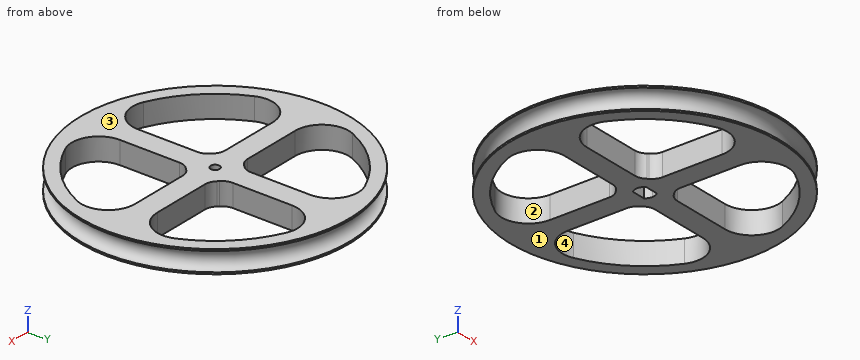
```python
from build123d import *

# Parameters (mm, degrees)
BOSS_EXTRUDE1_START = -6.35
SKETCH3_W           = 6.35
SKETCH3_H           = 6.35
BOSS_EXTRUDE1_DEPTH = 6.35
FILLET1_R           = 7.62
FILLET2_R           = 3.81
BOSS_EXTRUDE2_START = -1.5875
SKETCH4_R           = 1.27
BOSS_EXTRUDE2_DEPTH = 1.5875


with BuildPart() as part:
    # Sketch2 → Revolve1 (revolve)
    with BuildSketch(Plane(origin=(0, 0, 0), x_dir=(1, 0, 0), z_dir=(0, 1, 0))):
        with BuildLine():
            ThreePointArc((38.1, 2.667), (35.433, 0), (38.1, -2.667))
            Line((38.1, -2.667), (38.1, -3.175))
            Line((38.1, -3.175), (34.29, -3.175))
            Line((34.29, -3.175), (34.29, 3.175))
            Line((34.29, 3.175), (38.1, 3.175))
            Line((38.1, 3.175), (38.1, 2.667))
        make_face()
    revolve(axis=Axis((0, 0, 2.667), (0, 0, -1)))

    # Sketch3 → Boss-Extrude1 (add)
    # profile 1 of 19: a face of its own
    with BuildSketch(Plane.XY.offset(3.175).offset(BOSS_EXTRUDE1_START)):
        with BuildLine():
            ThreePointArc((-34.142692849, 3.175), (-34.29, 0), (-34.142692849, -3.175))
            Line((-34.142692849, -3.175), (-5.645432136, -3.175))
            ThreePointArc((-5.645432136, -3.175), (-6.477, 0), (-5.645432136, 3.175))
            Line((-5.645432136, 3.175), (-34.142692849, 3.175))
        make_face()
    # profile 2 of 19: a face of its own
    with BuildSketch(Plane.XY.offset(3.175).offset(BOSS_EXTRUDE1_START)):
        with BuildLine():
            Line((5.645432136, -3.175), (34.142692849, -3.175))
            ThreePointArc((34.142692849, -3.175), (34.253153415, -1.589207695), (34.29, 0))
            ThreePointArc((34.29, 0), (34.253153415, 1.589207695), (34.142692849, 3.175))
            Line((34.142692849, 3.175), (5.645432136, 3.175))
            ThreePointArc((5.645432136, 3.175), (6.265660099, 1.641046169), (6.477, 0))
            ThreePointArc((6.477, 0), (6.265660099, -1.641046169), (5.645432136, -3.175))
        make_face()
    # profile 3 of 19: a face of its own
    with BuildSketch(Plane.XY.offset(3.175).offset(BOSS_EXTRUDE1_START)):
        with BuildLine():
            ThreePointArc((-5.645432136, 3.175), (-6.477, 0), (-5.645432136, -3.175))
            Line((-5.645432136, -3.175), (-3.175, -3.175))
            Line((-3.175, -3.175), (-3.175, 3.175))
            Line((-3.175, 3.175), (-5.645432136, 3.175))
        make_face()
    # profile 4 of 19: a face of its own
    with BuildSketch(Plane.XY.offset(3.175).offset(BOSS_EXTRUDE1_START)):
        with BuildLine():
            Line((-3.175, 5.645432136), (-3.175, 3.175))
            Line((-3.175, 3.175), (3.175, 3.175))
            Line((3.175, 3.175), (3.175, 5.645432136))
            ThreePointArc((3.175, 5.645432136), (0, 6.477), (-3.175, 5.645432136))
        make_face()
    # profile 5 of 19: a face of its own
    with BuildSketch(Plane.XY.offset(3.175).offset(BOSS_EXTRUDE1_START)):
        with BuildLine():
            Line((-3.175, -5.645432136), (-3.175, -34.142692849))
            ThreePointArc((-3.175, -34.142692849), (0, -34.29), (3.175, -34.142692849))
            Line((3.175, -34.142692849), (3.175, -5.645432136))
            ThreePointArc((3.175, -5.645432136), (0, -6.477), (-3.175, -5.645432136))
        make_face()
    # profile 6 of 19: a face of its own
    with BuildSketch(Plane.XY.offset(3.175).offset(BOSS_EXTRUDE1_START)):
        with BuildLine():
            ThreePointArc((3.175, 34.142692849), (0, 34.29), (-3.175, 34.142692849))
            Line((-3.175, 34.142692849), (-3.175, 5.645432136))
            ThreePointArc((-3.175, 5.645432136), (0, 6.477), (3.175, 5.645432136))
            Line((3.175, 5.645432136), (3.175, 34.142692849))
        make_face()
    # profile 7 of 19: a face of its own
    with BuildSketch(Plane.XY.offset(3.175).offset(BOSS_EXTRUDE1_START)):
        with BuildLine():
            ThreePointArc((-3.175, 5.645432136), (-4.579930622, 4.579930622), (-5.645432136, 3.175))
            Line((-5.645432136, 3.175), (-3.175, 3.175))
            Line((-3.175, 3.175), (-3.175, 5.645432136))
        make_face()
    # profile 8 of 19: a face of its own
    with BuildSketch(Plane.XY.offset(3.175).offset(BOSS_EXTRUDE1_START)):
        with BuildLine():
            Line((3.175, 5.645432136), (3.175, 3.175))
            Line((3.175, 3.175), (5.645432136, 3.175))
            ThreePointArc((5.645432136, 3.175), (4.579930622, 4.579930622), (3.175, 5.645432136))
        make_face()
    # profile 9 of 19: a face of its own
    with BuildSketch(Plane.XY.offset(3.175).offset(BOSS_EXTRUDE1_START)):
        with BuildLine():
            Line((3.175, 3.175), (3.175, -3.175))
            Line((3.175, -3.175), (5.645432136, -3.175))
            ThreePointArc((5.645432136, -3.175), (6.265660099, -1.641046169), (6.477, 0))
            ThreePointArc((6.477, 0), (6.265660099, 1.641046169), (5.645432136, 3.175))
            Line((5.645432136, 3.175), (3.175, 3.175))
        make_face()
    # profile 10 of 19: a face of its own
    with BuildSketch(Plane.XY.offset(3.175).offset(BOSS_EXTRUDE1_START)):
        with BuildLine():
            ThreePointArc((-34.142692849, 3.175), (-34.29, 0), (-34.142692849, -3.175))
            Line((-34.142692849, -3.175), (-5.645432136, -3.175))
            ThreePointArc((-5.645432136, -3.175), (-6.477, 0), (-5.645432136, 3.175))
            Line((-5.645432136, 3.175), (-34.142692849, 3.175))
        make_face()
    # profile 11 of 19: a face of its own
    with BuildSketch(Plane.XY.offset(3.175).offset(BOSS_EXTRUDE1_START)):
        with BuildLine():
            Line((5.645432136, -3.175), (34.142692849, -3.175))
            ThreePointArc((34.142692849, -3.175), (34.253153415, -1.589207695), (34.29, 0))
            ThreePointArc((34.29, 0), (34.253153415, 1.589207695), (34.142692849, 3.175))
            Line((34.142692849, 3.175), (5.645432136, 3.175))
            ThreePointArc((5.645432136, 3.175), (6.265660099, 1.641046169), (6.477, 0))
            ThreePointArc((6.477, 0), (6.265660099, -1.641046169), (5.645432136, -3.175))
        make_face()
    # profile 12 of 19: a face of its own
    with BuildSketch(Plane.XY.offset(3.175).offset(BOSS_EXTRUDE1_START)):
        with BuildLine():
            Line((-3.175, -5.645432136), (-3.175, -34.142692849))
            ThreePointArc((-3.175, -34.142692849), (0, -34.29), (3.175, -34.142692849))
            Line((3.175, -34.142692849), (3.175, -5.645432136))
            ThreePointArc((3.175, -5.645432136), (0, -6.477), (-3.175, -5.645432136))
        make_face()
    # profile 13 of 19: a face of its own
    with BuildSketch(Plane.XY.offset(3.175).offset(BOSS_EXTRUDE1_START)):
        with BuildLine():
            ThreePointArc((3.175, 34.142692849), (0, 34.29), (-3.175, 34.142692849))
            Line((-3.175, 34.142692849), (-3.175, 5.645432136))
            ThreePointArc((-3.175, 5.645432136), (0, 6.477), (3.175, 5.645432136))
            Line((3.175, 5.645432136), (3.175, 34.142692849))
        make_face()
    # profile 14 of 19: a face of its own
    with BuildSketch(Plane.XY.offset(3.175).offset(BOSS_EXTRUDE1_START)):
        with BuildLine():
            Line((3.175, -3.175), (-3.175, -3.175))
            Line((-3.175, -3.175), (-3.175, -5.645432136))
            ThreePointArc((-3.175, -5.645432136), (0, -6.477), (3.175, -5.645432136))
            Line((3.175, -5.645432136), (3.175, -3.175))
        make_face()
    # profile 15 of 19: a face of its own
    with BuildSketch(Plane.XY.offset(3.175).offset(BOSS_EXTRUDE1_START)):
        with BuildLine():
            Line((-3.175, -3.175), (-5.645432136, -3.175))
            ThreePointArc((-5.645432136, -3.175), (-4.579930622, -4.579930622), (-3.175, -5.645432136))
            Line((-3.175, -5.645432136), (-3.175, -3.175))
        make_face()
    # profile 16 of 19: a face of its own
    with BuildSketch(Plane.XY.offset(3.175).offset(BOSS_EXTRUDE1_START)):
        with BuildLine():
            Line((5.645432136, -3.175), (3.175, -3.175))
            Line((3.175, -3.175), (3.175, -5.645432136))
            ThreePointArc((3.175, -5.645432136), (4.579930622, -4.579930622), (5.645432136, -3.175))
        make_face()
    # profile 17 of 19: a face of its own
    with BuildSketch(Plane.XY.offset(3.175).offset(BOSS_EXTRUDE1_START)):
        Rectangle(SKETCH3_W, SKETCH3_H)
        with BuildLine():
            ThreePointArc((-1.929188106, 1.8415), (0, 2.667), (1.929188106, 1.8415))
            ThreePointArc((1.929188106, 1.8415), (2.475685125, 0.991903302), (2.667, 0))
            ThreePointArc((2.667, 0), (2.475685125, -0.991903302), (1.929188106, -1.8415))
            ThreePointArc((1.929188106, -1.8415), (0, -2.667), (-1.929188106, -1.8415))
            ThreePointArc((-1.929188106, -1.8415), (-2.667, 0), (-1.929188106, 1.8415))
        make_face(mode=Mode.SUBTRACT)
    # profile 18 of 19: a face of its own
    with BuildSketch(Plane.XY.offset(3.175).offset(BOSS_EXTRUDE1_START)):
        with BuildLine():
            Line((-1.929188106, 1.8415), (1.929188106, 1.8415))
            ThreePointArc((1.929188106, 1.8415), (0, 2.667), (-1.929188106, 1.8415))
        make_face()
    # profile 19 of 19: a face of its own
    with BuildSketch(Plane.XY.offset(3.175).offset(BOSS_EXTRUDE1_START)):
        with BuildLine():
            Line((1.929188106, -1.8415), (-1.929188106, -1.8415))
            ThreePointArc((-1.929188106, -1.8415), (0, -2.667), (1.929188106, -1.8415))
        make_face()
    extrude(amount=BOSS_EXTRUDE1_DEPTH)

    # Fillet1
    fillet1_edges = [part.edges().sort_by_distance(p)[0] for p in [
        (34.142692849, -3.175, 0),
        (34.142692849, 3.175, 0),
        (3.175, 34.142692849, 0),
        (-3.175, 34.142692849, 0),
        (-34.142692849, 3.175, 0),
        (-34.142692849, -3.175, 0),
        (-3.175, -34.142692849, 0),
        (3.175, -34.142692849, 0),
    ]]
    fillet(fillet1_edges, radius=FILLET1_R)

    # Fillet2
    fillet2_edges = [part.edges().sort_by_distance(p)[0] for p in [
        (5.645432136, 3.175, 0),
        (3.175, 5.645432136, 0),
        (-3.175, 5.645432136, 0),
        (-5.645432136, 3.175, 0),
        (-5.645432136, -3.175, 0),
        (-3.175, -5.645432136, 0),
        (3.175, -5.645432136, 0),
        (5.645432136, -3.175, 0),
    ]]
    fillet(fillet2_edges, radius=FILLET2_R)

    # Sketch4 → Boss-Extrude2 (add)
    with BuildSketch(Plane.XY.offset(3.175).offset(BOSS_EXTRUDE2_START)):
        with BuildLine():
            Line((1.929188106, 1.8415), (-1.929188106, 1.8415))
            ThreePointArc((-1.929188106, 1.8415), (-2.667, 0), (-1.929188106, -1.8415))
            Line((-1.929188106, -1.8415), (1.929188106, -1.8415))
            ThreePointArc((1.929188106, -1.8415), (2.667, 0), (1.929188106, 1.8415))
        make_face()
        Circle(SKETCH4_R, mode=Mode.SUBTRACT)
    extrude(amount=BOSS_EXTRUDE2_DEPTH)


solid = part.part
```
Could you check a few things on this model? Use its own coordinates, in mm. Face numbers are marked on the shaded views. A direction names the side the tool comes from. Round coordinates to 2 decimals unless told otherwise and drop trailing zeros. Loops run counter-clockwise (first coordinate to the right, second up) from the corner with the lowest first, then second, coordinate; pieces in that order, holes last. Notation, with made-up numbers: (84, 66.5) - (128, 66.5) arc R21 ccw to (128, 94.5) - close; hole circle Ø10 at (25.25, -15.5). An arc over 180 degrees is marked (long way). Answer in a Markdown table with one row per item. Add a question column.
(1) If we mould it in two halves opening along Y, with no side actions, what happens to the marked faces 3 and 4? For each: pulls with the +Y half, pulls with the -Y half, needs draft (parallel to the pull), parting line crosses it, or undercut.
(2) I need wall thicknesses on line 1 along Y through (x, z) = (6, 0.5); line 2 along Y through (x, z) = (-27, -2.75); line 3 along X through (y, z) = (8, -2) (3 decimals). Which ranges of each line are inside material? Lowest first, please.
(3) If we section it at A-A (x = 0): Please give me the cut outline in (y, z) (1 decimal), plus the area to 3 significant figures.
(4) If we section it at B-B (z = 0): State how many separate pieces and enclosed holes the cut face has, plus the area to 3 significant figures.
(5) For the marked faces 1 and 2, which set-ups out of +Z, -Z, +X, -X, +Y, -Y let a thin tool reach every point of the face, with its end or its side?
(6) I'm going to push flat-ended pins straight in: pin 1 (3.5 mm diameter, centred on x = 0, y = 0, fed in from -Z); pin 2 (1.9 mm diameter, centred on x = -13, z = -0.5, fed in from -Y); pin 3 (1.9 mm diameter, centred on y = -15, z = 1.5, fed in from -X); pin 4 (4 mm diameter, centred on x = 0.5, y = -0.5, fed in from -Z) (3 decimals). Where does each tip first touch, or does it pass through?
Model answer:
| question | item | result |
|---|---|---|
| 1 | face 3 | needs draft |
| 1 | face 4 | undercut |
| 2 | line 1 | y = -34.97 to -30.31, -3.51 to 3.51, 30.31 to 34.97 |
| 2 | line 2 | y = -26.88 to -21.14, -3.64 to 3.64, 21.14 to 26.88 |
| 2 | line 3 | x = -35.444 to -31.477, -3.175 to 3.175, 31.477 to 35.444 |
| 3 | outline | (-38.1, -3.2) - (-1.8, -3.2) - (-1.8, 1.6) - (-1.3, 1.6) - (-1.3, 3.2) - (-38.1, 3.2) - (-38.1, 2.7) arc R2.7 cw to (-38.1, -2.7) - close; (1.3, 1.6) - (1.8, 1.6) - (1.8, -3.2) - (38.1, -3.2) - (38.1, -2.7) arc R2.7 cw to (38.1, 2.7) - (38.1, 3.2) - (1.3, 3.2) - close |
| 3 | area | 440 mm² |
| 4 | separate pieces | 1 |
| 4 | enclosed holes | 5 |
| 4 | area | 1,270 mm² |
| 5 | face 1 | -Z, +X, -X, +Y, -Y |
| 5 | face 2 | +Z, -Z |
| 6 | pin 1 | stops at z = 1.59 |
| 6 | pin 2 | stops at y = -33.52 |
| 6 | pin 3 | stops at x = -33.91 |
| 6 | pin 4 | stops at z = -3.175 |
